Geometry: final body of the model. Coordinates: model frame, mm. A direction names the side the tool comes from. Round coordinates to 2 decimals unless told otherwise and drop trailing zeros. Write each loop counter-clockwise with the first axis right and the second up, starting at its lowest first coordinate (ties: lowest second). Pieces come first, ordered by that corner, then holes. Notation, with made-up numbers: (76, -14.75) - (135, -14.75) arc R14 ccw to (135, 4.25) - close; hole circle Ø2 at (74.25, 1.5). An arc over 180 degrees is marked (long way). Use a Markdown table: item, result. Add a question column.
```python
from build123d import *

# Parameters (mm, degrees)
F0_R     = 74
F0_R_2   = 7.25
F0_R_3   = 32.75
F1_DEPTH = 3
F2_R     = 81
F2_R_2   = 74
F3_DEPTH = 40.5
F4_R     = 135
F4_R_2   = 81
F5_DEPTH = 13.8


with BuildPart() as f1:
    # F0 (on Front) → F1 (new body)
    with BuildSketch(Plane.XZ):
        Circle(F0_R)
        with Locations((-32.3281888761, -44.4959346906)):
            Circle(F0_R_2, mode=Mode.SUBTRACT)
        with Locations((32.3281888761, -44.4959346906)):
            Circle(F0_R_2, mode=Mode.SUBTRACT)
        with Locations((-52.3081083962, 16.9959346906)):
            Circle(F0_R_2, mode=Mode.SUBTRACT)
        Circle(F0_R_3, mode=Mode.SUBTRACT)
        with Locations((52.3081083962, 16.9959346906)):
            Circle(F0_R_2, mode=Mode.SUBTRACT)
        with Locations((0, 55)):
            Circle(F0_R_2, mode=Mode.SUBTRACT)
    extrude(amount=F1_DEPTH)

    # F2 (on face) → F3 (join)
    with BuildSketch(Plane(origin=(0, 0, 0), x_dir=(-1, 0, 0), z_dir=(0, 1, 0))):
        Circle(F2_R)
        Circle(F2_R_2, mode=Mode.SUBTRACT)
    extrude(amount=-F3_DEPTH)

    # F4 (on face) → F5 (join)
    with BuildSketch(Plane.XZ.offset(40.5)):
        Circle(F4_R)
        Circle(F4_R_2, mode=Mode.SUBTRACT)
    extrude(amount=-F5_DEPTH)


solid = f1.part
```
1) Material intervals for L1, parallel to Z at x = 0, y = -13; L2, parallel to Y at x = 5, z = -65.5; L3, parallel to Y at x = 103.5, z = 51.5, sorted ascending. Write a range as from..to.
2) Section C-C, the plane y = -10. Return the cut outline in (x, z).
3) Set-up query: faces 4 (the flat face through (58, -26.7, -58)), 5 (the cylindrical face through (3.35, -1.48, 48.57)), 6 (the flat face through (32, -3, -15)). Return all of +Z, -Z, +X, -X, +Y, -Y with unobstructed straight access to the full face (end or side cutting, diameter ignored); none if empty.
4) Pin query (flat end, axial travel): P1, Ø6, axis at x = 41.5, y = -20.5, coming from the -Z side; P2, Ø5, axis at x = 5.5, y = -9, coming from the +Z side; P3, Ø6, axis at y = -26.5, z = -25, coming from the -X side. Return the tip coordinate at first contact, or that it passes through.
5) Section D-D, the plane z = 55. Return the cut outline in (x, y).
6) Draft query along X for faces 1 (the flat face through (1, 0, -35)), 2 (the cylindrical face through (-43.545, -13.163, 68.3)), 3 (the cylindrical face through (50.736, -1.479, 9.918)). Return one class per face: released by +X, released by -X, zero draft, split by the parting line, or undercut.
7) Section B-B, the plane z = 0. Return the cut outline in (x, y), then the cut area to 3 significant figures.
8) Section A-A, the plane x = 0. Return the cut outline in (y, z), then the cut area to 3 significant figures.
Output values:
| question | item | result |
|---|---|---|
| 1 | L1 | z = -81..-74, 74..81 |
| 1 | L2 | y = -3..0 |
| 1 | L3 | y = -40.5..-26.7 |
| 2 | outline | circle Ø162 at (0, 0); hole circle Ø148 at (0, 0) |
| 3 | face 4 | +Y |
| 3 | face 5 | +Y, -Y |
| 3 | face 6 | -Y |
| 4 | P1 | stops at z = -71.27 |
| 4 | P2 | stops at z = 80.94 |
| 4 | P3 | stops at x = -133.19 |
| 5 | outline | (-123.29, -40.5) - (-49.51, -40.5) - (-49.51, -3) - (-7.25, -3) - (-7.25, 0) - (-59.46, 0) - (-59.46, -26.7) - (-123.29, -26.7) - close; (7.25, -3) - (49.51, -3) - (49.51, -40.5) - (123.29, -40.5) - (123.29, -26.7) - (59.46, -26.7) - (59.46, 0) - (7.25, 0) - close |
| 6 | face 1 | zero draft |
| 6 | face 2 | split by the parting line |
| 6 | face 3 | undercut |
| 7 | outline | (-135, -40.5) - (-74, -40.5) - (-74, -3) - (-32.75, -3) - (-32.75, 0) - (-81, 0) - (-81, -26.7) - (-135, -26.7) - close; (32.75, -3) - (74, -3) - (74, -40.5) - (135, -40.5) - (135, -26.7) - (81, -26.7) - (81, 0) - (32.75, 0) - close |
| 7 | area | 2,300 mm^2 |
| 8 | outline | (-40.5, -135) - (-26.7, -135) - (-26.7, -81) - (0, -81) - (0, -32.75) - (-3, -32.75) - (-3, -74) - (-40.5, -74) - close; (-40.5, 74) - (-3, 74) - (-3, 62.25) - (0, 62.25) - (0, 81) - (-26.7, 81) - (-26.7, 135) - (-40.5, 135) - close; (-3, 32.75) - (0, 32.75) - (0, 47.75) - (-3, 47.75) - close |
| 8 | area | 2,260 mm^2 |
